Autodesk Inventor part; units mm, degrees
ref_plane "YZ Plane" through (0, 0, 0) normal (1, 0, 0) x (0, 1, 0)
ref_plane "XZ Plane" through (0, 0, 0) normal (0, 1, 0) x (-1, 0, 0)
ref_plane "XY Plane" through (0, 0, 0) normal (0, 0, 1) x (1, 0, 0)
sketch "Sketch1" plane through (0, 0, 0) normal (0, 0, 1) x (1, 0, 0)
  circle A0 centre (-15.5, -15.5) radius 1.75
  circle A1 centre (15.5, -15.5) radius 1.75
  circle A2 centre (-15.5, 15.5) radius 1.75
  circle A3 centre (15.5, 15.5) radius 1.75
  circle A4 centre (0, 0) radius 12.5
  line L0 (-21.5, 21.5) -> (21.5, 21.5)
  line L1 (21.5, -21.5) -> (-21.5, -21.5)
  line L2 (-21.5, 21.5) -> (21.5, -21.5) construction
  line L3 (21.5, 21.5) -> (-21.5, -21.5) construction
  line L4 (-21.5, -21.5) -> (21.5, -21.5)
  line L5 (-21.5, 21.5) -> (-21.5, -21.5)
  line L6 (21.5, 21.5) -> (21.5, -21.5)
  line L7 (-21.5, 21.5) -> (21.5, 21.5)
  line L8 (21.5, 21.5) -> (21.5, 26.5)
  line L9 (21.5, 26.5) -> (-21.5, 26.5)
  line L10 (-21.5, 26.5) -> (-21.5, 21.5)
  line L11 (0, 0) -> (-7.0913, 0)
  line L12 (21.5, -21.5) -> (21.5, -26.5)
  line L13 (21.5, -26.5) -> (-21.5, -26.5)
  line L14 (-21.5, -26.5) -> (-21.5, -21.5)
  point P0 (0, 26.5)
  point P1 (0, -26.5)
  point P2 (21.5, 21.5)
  dimension "d0" = 3.5
  dimension "d1" = 31
  dimension "d2" = 25
  dimension "d3" = 43
  dimension "d4" = 43
  dimension "d6" = 15.5
  dimension "d7" = 43
  dimension "d8" = 5
extrude "face" add sketch "Sketch1" against normal blind 5
extrude "length" add sketch "Sketch1" along normal blind 55 contours L10 L9 L8 L0 | L1 L12 L13 L14
sketch "Sketch2" plane through (0, 0, 55) normal (0, 0, 1) x (1, 0, 0)
  line L0 (-21.5, -21.5) -> (21.5, -21.5)
  line L1 (21.5, -21.5) -> (21.5, 21.5)
  line L2 (21.5, 21.5) -> (-21.5, 21.5)
  line L3 (-21.5, 21.5) -> (-21.5, -21.5)
  circle A0 centre (15.5, 15.5) radius 1.75
  circle A1 centre (-15.5, 15.5) radius 1.75
  circle A2 centre (-15.5, -15.5) radius 1.75
  circle A3 centre (15.5, -15.5) radius 1.75
  circle A4 centre (0, 0) radius 12.5
  line L4 (-21.5, 26.5) -> (-21.5, 21.5)
  line L5 (-21.5, 21.5) -> (21.5, 21.5)
  line L6 (21.5, 21.5) -> (21.5, 26.5)
  line L7 (21.5, 26.5) -> (-21.5, 26.5)
  line L8 (21.5, -26.5) -> (21.5, -21.5)
  line L9 (21.5, -21.5) -> (-21.5, -21.5)
  line L10 (-21.5, -21.5) -> (-21.5, -26.5)
  line L11 (-21.5, -26.5) -> (21.5, -26.5)
  line L12 (-21.5, 26.5) -> (21.5, 26.5)
  line L13 (21.5, 26.5) -> (21.5, 35.5)
  line L14 (21.5, 35.5) -> (-21.5, 35.5)
  line L15 (-21.5, 35.5) -> (-21.5, 26.5)
  line L16 (0, 0) -> (-5.3455, 0)
  line L17 (21.5, -26.5) -> (21.5, -35.5)
  line L18 (21.5, -35.5) -> (-21.5, -35.5)
  line L19 (-21.5, -35.5) -> (-21.5, -26.5)
  line L20 (-21.5, -26.5) -> (21.5, -26.5)
  circle A5 centre (0, -31) radius 2.25
  circle A6 centre (0, 31) radius 2.25
  point P0 (-21.5, -31)
  dimension "d13" = 9
  dimension "d19" = 4.5
extrude "mount" add sketch "Sketch2" along normal blind 5 contours L0 L8 L11 L10 | L4 L7 L6 L2 | L11 L17 L18 L19 | L15 L14 L13 L7
fillet "Fillet3" radius 2 2 edges at (0, -21.5, 0) (0, 21.5, 0)
fillet "Fillet4" radius 2 2 edges at (0, 21.5, 60) (0, -21.5, 60)
fillet "Fillet5" radius 2 6 edges at (0, -26.5, -5) (0, 26.5, -5) (0, 35.5, 55) (0, 35.5, 60) (0, -35.5, 55) (0, -35.5, 60)
properties part number "motor_holder_V4"
Geometry: final body of the model. Coordinates: model frame, mm. A direction names the side the tool comes from. Round coordinates to 2 decimals unless told otherwise and drop trailing zeros. Write each loop counter-clockwise with the first axis right and the second up, starting at its lowest first coordinate (ties: lowest second). Pieces come first, ordered by that corner, then holes. Notation, with made-up numbers: (46, -8) -> (55, -8) arc R8 ccw to (55, 2) -> close; hole circle Ø1 at (-31, 26). An arc over 180 degrees is marked (long way). Use CSV: the item, a comma, the result in double quotes. Start each with the question number.
Q1. Reachability of faces 1 (the face through (0, 28, 55)), 2 (the face through (-0.3, -20.9, 0.57)), 3 (the face through (0, -28, 55)) from +Z, -Z, +X, -X, +Y, -Y: full face, straight path, thin tool, end or side. Return the list, or none.
Q2. Pull-direction query (X, two-part tool) for faces 4 (the face through (21.5, -24, 25)), 5 (the face through (-0.3, -25.9, -4.43)), 6 (the face through (-1.786, 32.369, 57.465)); classes: pulls with the +X half, pulls with the -X half, needs draft (parallel to the pull), parting line crosses it, or undercut.
Q3. First-contact query: pin 1 Ø8 at (x, z) = (14, 13) entering from +Y; pin 2 Ø7.5 at (x, y) = (9, 30) entering from -Z; pin 3 Ø2 at (x, y) = (15.5, 15.5) entering from -Z; pin 4 Ø3 at (x, z) = (-3, 25.5) entering from -Y. Flat tips, straight axial feed; report the tip coordinate or a pass-through.
Q4. Line query: L1, parallel to Y at x = -15.5, z = -3.2; L2, parallel to Y at x = 0, z = 58; L3, parallel to Y at x = 15.5, z = -3.65. Output: solid intervals per line, ascending.
Q5. Section C-C (z = 8). Return loops of the section in (x, y).
Q6. Section D-D (y = 31). Return loops of the section in (x, z).
Q7. Section B-B (x = 0). Give the number of separate pieces and of enclosed holes in the cut face, plus the area to 3 significant figures.
Q8. Section A-A (y = -15.5). Return loops of the section in (x, z).
Result sheet:
1,face 1,"-Z, +X, -X, +Y"
1,face 2,"+Z, +X, -X"
1,face 3,"-Z, +X, -X, -Y"
2,face 4,"pulls with the +X half"
2,face 5,"needs draft"
2,face 6,"undercut"
3,pin 1,"y = 26.5"
3,pin 2,"z = -3.97"
3,pin 3,"through"
3,pin 4,"y = -26.5"
4,L1,"-26.49 to -17.25, -13.75 to 13.75, 17.25 to 26.49"
4,L2,"-35.5 to -33.25, -28.75 to -21.5, 21.5 to 28.75, 33.25 to 35.5"
4,L3,"-26.39 to -17.25, -13.75 to 13.75, 17.25 to 26.39"
5,outline,"(-21.5, -26.5) -> (21.5, -26.5) -> (21.5, -21.5) -> (-21.5, -21.5) -> close; (-21.5, 21.5) -> (21.5, 21.5) -> (21.5, 26.5) -> (-21.5, 26.5) -> close"
6,outline,"(-21.5, 55) -> (-2.25, 55) -> (-2.25, 60) -> (-21.5, 60) -> close; (2.25, 55) -> (21.5, 55) -> (21.5, 60) -> (2.25, 60) -> close"
7,separate pieces,"4"
7,enclosed holes,"0"
7,area,"780 mm²"
8,outline,"(-21.5, -5) -> (-17.25, -5) -> (-17.25, 0) -> (-21.5, 0) -> close; (-13.75, -5) -> (13.75, -5) -> (13.75, 0) -> (-13.75, 0) -> close; (17.25, -5) -> (21.5, -5) -> (21.5, 0) -> (17.25, 0) -> close"
